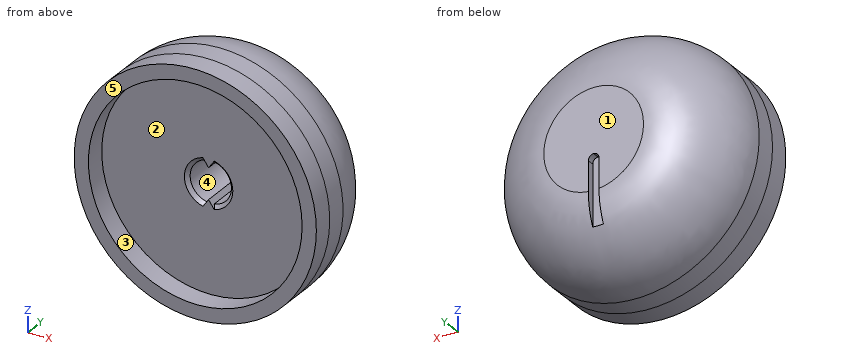
Autodesk Inventor part; units mm, degrees
ref_plane "YZ Plane" through (0, 0, 0) normal (1, 0, 0) x (0, 1, 0)
ref_plane "XZ Plane" through (0, 0, 0) normal (0, 1, 0) x (-1, 0, 0)
ref_plane "XY Plane" through (0, 0, 0) normal (0, 0, 1) x (1, 0, 0)
sketch "Sketch1" plane through (0, 0, 0) normal (0, 1, 0) x (-1, 0, 0)
  circle A0 centre (0, 0) radius 17
  dimension "d0" = 34
extrude "Extrusion1" add sketch "Sketch1" along normal blind 13
chamfer "Chamfer1" distance 4 angle 45 1 edges at (17, 13, 0)
sketch "Sketch2" plane through (0, 13, 0) normal (0, 1, 0) x (1, 0, 0)
  line L0 (0.75, 2) -> (-0.75, 2)
  line L1 (-0.75, 2) -> (-0.75, 12)
  line L2 (-0.75, 12) -> (0.75, 12)
  line L3 (0.75, 12) -> (0.75, 2)
  circle A0 centre (0, 0) radius 17
  dimension "d6" = 1.5
  dimension "d7" = 10
  dimension "d8" = 2
  dimension "d9" = 16.25
extrude "Extrusion2" cut sketch "Sketch2" against normal blind 1 contours L0 L1 L2 L3
fillet "Fillet1" radius 0.75 4 edges at (0.75, 12.5, -12) (-0.75, 12.5, -12) (-0.75, 12.5, -2) (0.75, 12.5, -2)
sketch "Sketch3" plane through (0, 0, 0) normal (0, -1, 0) x (1, 0, 0)
  circle A0 centre (0, 0) radius 2.9
  line L0 (0, 0) -> (3.3833, 0) construction
  line L1 (0, 0) -> (3.3833, 0) construction
  line L2 (0, 0) -> (2.9, 0) construction
  line L3 (0, 0) -> (2.9, 0) construction
  line L4 (0, 0) -> (2.9, 0) construction
  line L5 (0, 0) -> (-0.4833, -2.8594)
  line L6 (0, 0) -> (2.9, 0) construction
  line L7 (-0.4833, -2.8594) -> (0.4833, -2.8594)
  line L8 (0, 0) -> (-0.4833, 2.8594)
  line L9 (0, 0) -> (2.9, 0) construction
  line L10 (-0.4833, 2.8594) -> (0.4833, 2.8594)
  line L11 (0.4833, 2.8594) -> (1.1703, 2.8594) construction
  line L12 (0.4833, 2.8594) -> (0, 2.1692)
  line L13 (0.4833, 2.8594) -> (1.326, 2.8594) construction
  line L14 (0, 2.1692) -> (-0.4833, 2.8594)
  line L15 (0.4833, -2.8594) -> (0, -2.1692)
  line L16 (0.4833, -2.8594) -> (1.326, -2.8594) construction
  line L17 (0, -2.1692) -> (-0.4833, -2.8594)
  dimension "d13" = 5.8
  dimension "d50" = 99.594
  dimension "d52" = 99.594
  dimension "d54" = 125
  dimension "d55" = 125
extrude "Extrusion7" cut sketch "Sketch3" against normal blind 10.5 contours A0 L15 L17 L5 L8 L14 L12 | L8 L5 A0
sketch "Sketch5" plane through (0, 0, 0) normal (0, -1, 0) x (1, 0, 0)
  circle A0 centre (0, 0) radius 17
  circle A1 centre (0, 0) radius 15
extrude "Extrusion8" add sketch "Sketch5" along normal blind 3
chamfer "Chamfer2" distance 0.5 angle 45 2 edges at (-2.9, 0, 0) (2.9, 0, 0)
fillet "Fillet6" radius 10 2 edges at (13, 13, 0) (17, 9, 0)
properties part number "knob"
Can you work these out from the model? Positions are in its coordinate system, mm. Face numbers are marked on the shaded views. A direction names the side the tool comes from. Give positions to 0.01 mm unless a question says otherwise; leave off trailing zeros. Write each loop counter-clockwise with the first axis right and the second up, starting at its lowest first coordinate (ties: lowest second). Pieces come first, ordered by that corner, then holes. Notation, with made-up numbers: M -8,-36.5 L 36,-36.5 A19 cw 36,-2.5 Z; hole C 60,37 d9. An arc over 180 degrees is marked long. Answer in a Markdown table with one row per item. Add a question column.
Item 1: Please list where these lines run through material, in increasing order: L1, parallel to Z at x = 0, y = -1.8; L2, parallel to X at y = 4.5, z = 7.5; L3, parallel to Y at x = -13, z = -9.
Item 2: Imagine slicing it at A-A, the plane y = -1.5. Write out the boundary of the cut face in (x, z).
Item 3: For pin 1 Ø2 at (x, y) = (11.5, 2) entering from +Z; pin 2 Ø3 at (y, z) = (-0.5, -5) entering from +X; pin 3 Ø6 at (y, z) = (4, 0) entering from +X; pin 4 Ø2 at (y, z) = (0, 13) entering from -X, each with a flat end and sliding along its axis, tell me the tip position at first contact or that it passes through.
Item 4: We'd pull the mould along X, two halves only. Please class the marked faces 3, 4 and 5: released by +X, released by -X, zero draft, split by the parting line, or undercut.
Item 5: On a 3-axis mill with a long thin cutter (end or side, diameter ignored), from which of +Z, -Z, +X, -X, +Y, -Y can I reach the whole of each face in a straight line? I mean the marked faces 1 and 2. Say none if no direction works.
Evaluation:
| question | item | result |
|---|---|---|
| 1 | L1 | z = -17 to -15, 15 to 17 |
| 1 | L2 | x = -15.13 to 15.13 |
| 1 | L3 | y = -3 to 7.73 |
| 2 | outline | C 0,0 d34; hole C 0,0 d30 |
| 3 | pin 1 | stops at z = 13.37 |
| 3 | pin 2 | stops at x = 16.64 |
| 3 | pin 3 | stops at x = 17 |
| 3 | pin 4 | stops at x = -12.04 |
| 4 | face 3 | undercut |
| 4 | face 4 | undercut |
| 4 | face 5 | zero draft |
| 5 | face 1 | +Z, -Z, +X, -X, +Y |
| 5 | face 2 | -Y |
